The figure shows three views and two pictorial views of one solid part (mm, origin at its lowest corner). Answer the questions. A direction names the side the tool comes from. Give positions to 0.01 mm unless a question says otherwise; leave off trailing zeros. Write each loop counter-clockwise with the first axis right and the second up, starting at its lowest first coordinate (ties: lowest second). Pieces come first, ordered by that corner, then holes. Notation, with made-up numbers: (66, 48) - (106, 48) arc R27 cw to (106, 71) - close; hole circle Ø1 at (63, -14). An arc over 180 degrees is marked (long way). One line per question, with ' | ' between items. Start each with the question number.
1. Given P1, Ø0.9, axis at x = 10, y = 7.5, coming from the +Z side; P2, Ø3, axis at y = 9, z = 10.5, coming from the +X side; P3, Ø2, axis at y = 2, z = 3.5, coming from the -X side, each flat-ended and moving along its own axis, determine where each tip first touches the part or whether it passes through.
2. A cutting plane is placed at C-C (z = 4.5). Determine the outline of the cut face in (x, y).
3. A cutting plane is placed at B-B (y = 7.2). Determine the outline of the cut face in (x, z), then the cut area to 3 significant figures.
4. A cutting plane is placed at A-A (x = 7.2). Determine the outline of the cut face in (y, z), then the cut area to 3 significant figures.
5. For the marked faces 1 and 2, determine the directions among +Z, -Z, +X, -X, +Y, -Y from which every point of the face is accessible in a straight line to the end or side of a thin tool.
6. Find the intervals of material crossed by L1, parallel to Y at x = 4.2, z = 23.5; L2, parallel to X at y = 7, z = 15.25; L3, parallel to Z at x = 7.25, y = 14, in increasing order. Write a range as from..to.
7. A cutting plane is placed at D-D (z = 14.5). Determine the outline of the cut face in (x, y), then the cut area to 3 significant figures.
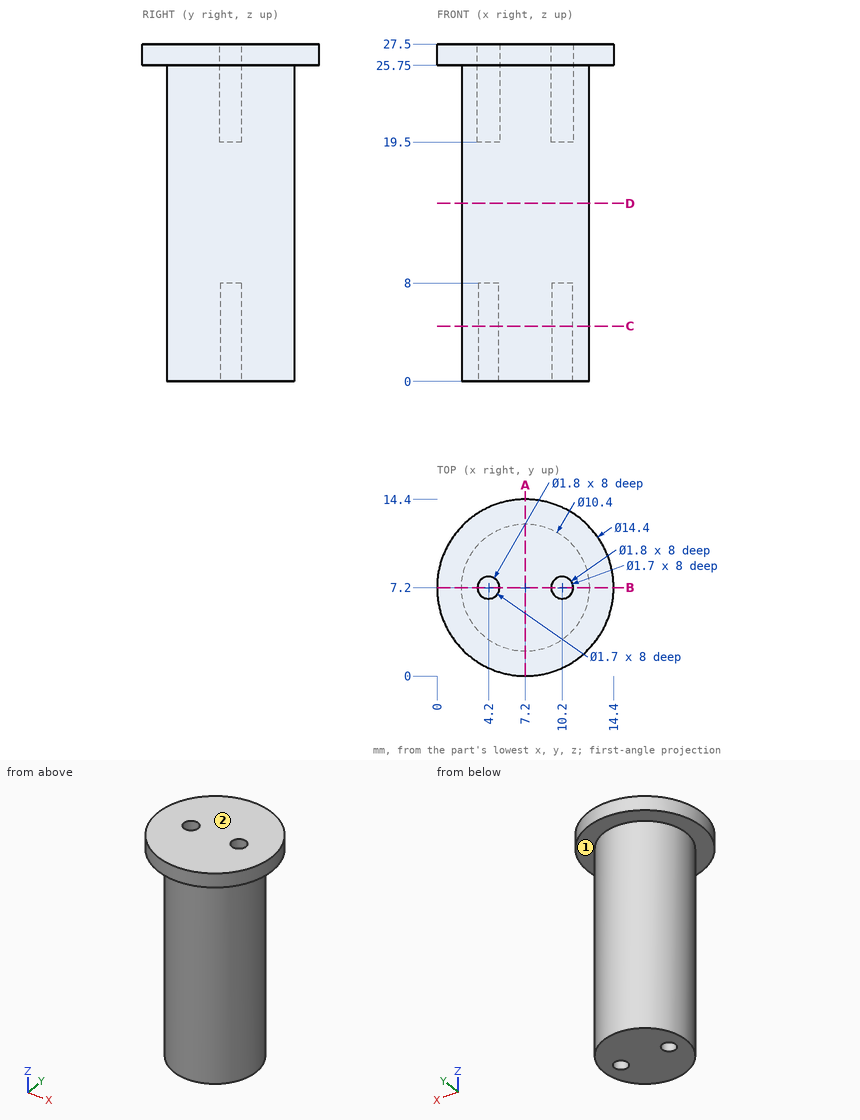
Determined:
1) P1: z = 19.5 | P2: x = 12.39 | P3: x = 4.13
2) outline: circle Ø10.4 at (7.2, 7.2); hole circle Ø1.7 at (4.2, 7.2); hole circle Ø1.7 at (10.2, 7.2)
3) outline: (0, 25.75) - (2, 25.75) - (2, 0) - (3.35, 0) - (3.35, 8) - (5.05, 8) - (5.05, 0) - (9.35, 0) - (9.35, 8) - (11.05, 8) - (11.05, 0) - (12.4, 0) - (12.4, 25.75) - (14.4, 25.75) - (14.4, 27.5) - (11.1, 27.5) - (11.1, 19.5) - (9.3, 19.5) - (9.3, 27.5) - (5.1, 27.5) - (5.1, 19.5) - (3.3, 19.5) - (3.3, 27.5) - (0, 27.5) - close | area: 237 mm2
4) outline: (0, 25.75) - (2, 25.75) - (2, 0) - (12.4, 0) - (12.4, 25.75) - (14.4, 25.75) - (14.4, 27.5) - (0, 27.5) - close | area: 293 mm2
5) face 1: -Z | face 2: +Z, +X, -X, +Y, -Y
6) L1: 2.95..6.3, 8.1..11.45 | L2: 2..12.4 | L3: 25.75..27.5
7) outline: circle Ø10.4 at (7.2, 7.2) | area: 84.9 mm2
